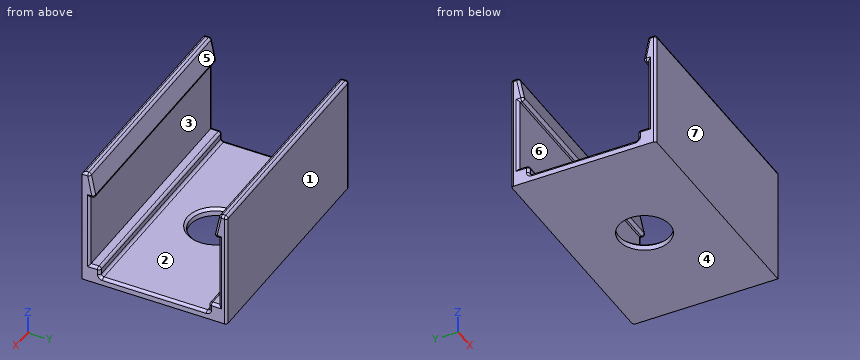
Autodesk Fusion 360 part; units mm, degrees
sketch "Sketch1" plane through (0, 0, 0) normal (0, 0, 1) x (1, 0, 0)
  line L0 (9, -5.65) -> (-9, -5.65)
  line L1 (-9, -5.65) -> (-9, 5.65)
  line L2 (-9, 5.65) -> (9, 5.65)
  line L3 (9, 5.65) -> (9, -5.65)
  line L4 (9, -5.65) -> (-9, 5.65) construction
  line L5 (-9, -5.65) -> (9, 5.65) construction
  line L6 (-9, 4.25) -> (9, 4.25)
  line L7 (-9, -4.25) -> (9, -4.25)
  line L8 (-9, 5.05) -> (9, 5.05)
  line L9 (-9, -5.05) -> (9, -5.05)
  circle A0 centre (0, 0) radius 2
  dimension "d1" = 18
  dimension "d2" = 11.3
  dimension "d5" = 1.4
  dimension "d6" = 1.4
  dimension "d9" = 0.6
  dimension "d10" = 0.6
  dimension "d21" = 4
extrude "Extrude1" add sketch "Sketch1" along normal blind 0.6
extrude "Extrude2" add sketch "Sketch1" along normal blind 1.4 contours L0 L1 L3 L9 | L1 L3 L7 L9 | L1 L3 L6 L8 | L1 L2 L3 L8
extrude "Extrude3" add sketch "Sketch1" along normal blind 9.2 contours L0 L1 L3 L9 | L1 L2 L3 L8
sketch "Sketch2" plane through (-9, 0, 0) normal (-1, 0, 0) x (0, -1, 0)
  line L0 (5.05, 1.4) -> (4.25, 1.4)
  line L1 (4.25, 1.4) -> (4.25, 0.6)
  line L2 (4.25, 0.6) -> (-4.25, 0.6)
  line L3 (-4.25, 0.6) -> (-4.25, 1.4)
  line L4 (-4.25, 1.4) -> (-5.05, 1.4)
  line L5 (-5.05, 1.4) -> (-5.05, 9.2)
  line L6 (-5.05, 9.2) -> (-5.65, 9.2)
  line L7 (-5.65, 9.2) -> (-5.65, 0)
  line L8 (-5.65, 0) -> (5.65, 0)
  line L9 (5.05, 9.2) -> (5.05, 1.4)
  line L10 (4.65, 7.2) -> (5.05, 7.2)
  line L11 (4.65, 7.2) -> (5.05, 9.2)
  line L12 (5.05, 7.2) -> (5.05, 9.2)
  line L13 (0, 0) -> (0, 9)
  line L14 (-4.65, 7.2) -> (-5.05, 9.2)
  line L15 (-5.05, 7.2) -> (-5.05, 9.2)
  line L16 (-4.65, 7.2) -> (-5.05, 7.2)
  point P0 (-5.05, 9.2)
extrude "Extrude4" add sketch "Sketch2" against normal blind 18 contours L9 L10 L11 L12 | L5 L14 L15 L16
fillet "Fillet1" radius 0.2 39 edges at (0, 4.65, 7.2) (0, -4.65, 7.2) (0, -4.25, 1.4) (0, 4.25, 1.4) (0, 4.25, 0.6) (0, -4.25, 0.6) (-9, 5.65, 4.6) (-9, 4.85, 8.2) (-9, 5.05, 4.3) (-9, 4.85, 7.2) (-9, -4.85, 7.2) (-9, -5.05, 4.3) (-9, -4.85, 8.2) (9, -4.85, 8.2) (9, -4.85, 7.2) (9, -5.05, 4.3) (9, 5.05, 4.3) (9, 4.85, 8.2) (9, 4.85, 7.2) (9, -4.65, 1.4) (9, 4.65, 1.4) (9, 4.25, 1) (9, -4.25, 1) (9, 0, 0.6) (-9, 0, 0.6) (-9, 4.65, 1.4) (-9, 4.25, 1) (-9, -4.25, 1) (-9, -4.65, 1.4) (-9, -5.65, 4.6) (-9, -5.35, 9.2) (0, -5.65, 9.2) (0, 5.65, 9.2) (0, 5.05, 9.2) (-9, 5.35, 9.2) (9, 5.35, 9.2) (9, -5.35, 9.2) (0, -5.05, 9.2) (9, 5.65, 4.6)
chamfer "Chamfer1" distance 0.2 angle 45 1 edges at (-1.8647, 0.7232, 0.6)
Part model, mm, in its own coordinate system. Face numbers are marked on the shaded views. A direction names the side the tool comes from. Round coordinates to 2 decimals unless told otherwise and drop trailing zeros. Order: outer loops, then holes, each group sorted by start corner. A loop starts at its lowest first (then second) coordinate and runs counter-clockwise, first axis right, second up. Notation, with made-up numbers: M 48.25,-33.75 L 87.25,-33.75 A15 cw 87.25,-19.75 Z; hole C -23,56 d9. An arc over 180 degrees is marked long. Put each result on its own line as item: value. Start each with the question number.
1. Drill centre lines: probe 1 along Y at (x, z) = (0, 0.35); probe 2 along Y at (x, z) = (4.5, 2.5); probe 3 along Z at (x, y) = (-5.25, -1.25). Where is each one in solid material? Low to high. Write a range as [from, to].
2. Slice it at D-D on x = 4.5. List the corners of the cut face in (y, z), then the cut area to 3 significant figures.
3. Two-plate mould, pull along Z, no slides. Class the marked faces 4, 5, 6 and 7: +Z half, -Z half, draft (parallel to the pull), parting line (faces both ways), or undercut.
4. Slice it at C-C on z = 3.75. List the corners of the cut face in (x, y), then the cut area to 3 significant figures.
5. Slice it at B-B on y = 0. List the corners of the cut face in (x, z).
6. Drop a flat-ended pin along its axis: pin 1 (5 mm diameter, centred on x = 0, y = 0, fed in from +Z). Give the stop position or say it passes through.
7. Tool access for the marked faces 1, 2 and 3: list every direction of +Z, -Z, +X, -X, +Y, -Y with a clear straight run to the whole face (end or side of a thin tool).
Findings:
1. probe 1: [-5.65, -2], [2, 5.65]
1. probe 2: [-5.65, -5.05], [5.05, 5.65]
1. probe 3: [0, 0.6]
2. outline: M -5.65,0 L 5.65,0 L 5.65,9 A0.2 ccw 5.45,9.2 L 5.21,9.2 A0.2 ccw 5.02,9.04 L 4.7,7.44 A0.2 ccw 4.89,7.2 L 5.05,7.2 L 5.05,1.4 L 4.45,1.4 A0.2 ccw 4.25,1.2 L 4.25,0.8 A0.2 cw 4.05,0.6 L -4.05,0.6 A0.2 cw -4.25,0.8 L -4.25,1.2 A0.2 ccw -4.45,1.4 L -5.05,1.4 L -5.05,7.2 L -4.89,7.2 A0.2 ccw -4.7,7.44 L -5.02,9.04 A0.2 ccw -5.21,9.2 L -5.45,9.2 A0.2 ccw -5.65,9 Z
2. area: 19.1 mm2
3. face 4: -Z half
3. face 5: +Z half
3. face 6: undercut
3. face 7: draft
4. outline: M -9,-5.45 A0.2 ccw -8.8,-5.65 L 9,-5.65 L 9,-5.25 A0.2 ccw 8.8,-5.05 L -8.8,-5.05 A0.2 ccw -9,-5.25 Z; M -9,5.25 A0.2 ccw -8.8,5.05 L 8.8,5.05 A0.2 ccw 9,5.25 L 9,5.45 A0.2 ccw 8.8,5.65 L -8.8,5.65 A0.2 ccw -9,5.45 Z
4. area: 21.5 mm2
5. outline: M -9,0 L -2,0 L -2,0.4 L -2.2,0.6 L -8.8,0.6 A0.2 ccw -9,0.4 Z; M 2,0 L 9,0 L 9,0.4 A0.2 ccw 8.8,0.6 L 2.2,0.6 L 2,0.4 Z
6. pin 1: z = 0.6
7. face 1: +Z, -Z, +X, -X, +Y
7. face 2: +Z, +X, -X
7. face 3: +X, -X
